```python
from build123d import *

# Parameters (mm, degrees)
SKETCH1_W                      = 276.225
SKETCH1_H                      = 98.425
BOSS_EXTRUDE1_DEPTH            = 6.35
F_5_16_0_332_DOWEL_HOLE1_D     = 7.9375
F_5_16_0_332_DOWEL_HOLE1_DEPTH = 6.35
SKETCH5_W                      = 12.7
SKETCH5_H                      = 12.7
CUT_EXTRUDE1_DEPTH             = 7.35
FILLET1_R                      = 3.175
FILLET2_R                      = 6.35
F_1_4_0_2500_DOWEL_HOLE1_D     = 6.35
F_1_4_0_2500_DOWEL_HOLE1_DEPTH = 6.35


with BuildPart() as part:
    # Sketch1 → Boss-Extrude1 (new body)
    with BuildSketch(Plane(origin=(0, 0, 0), x_dir=(1, 0, 0), z_dir=(0, 1, 0))):
        Rectangle(SKETCH1_W, SKETCH1_H)
    extrude(amount=BOSS_EXTRUDE1_DEPTH)

    # 5/16 (0.332) Dowel Hole1
    with Locations(Plane(origin=(0, 6.35, 0), x_dir=(1, 0, 0), z_dir=(0, 1, 0))):
        with Locations((-93.6625, 0), (93.6625, 0)):
            Hole(F_5_16_0_332_DOWEL_HOLE1_D / 2, depth=F_5_16_0_332_DOWEL_HOLE1_DEPTH)

    # Sketch5 → Cut-Extrude1 (cut, through all)
    with BuildSketch(Plane(origin=(0, 6.35, 0), x_dir=(1, 0, 0), z_dir=(0, 1, 0))):
        with Locations((-131.7625, 0)):
            Rectangle(SKETCH5_W, SKETCH5_H)
        with Locations((131.7625, 0)):
            Rectangle(SKETCH5_W, SKETCH5_H)
    extrude(amount=-CUT_EXTRUDE1_DEPTH, mode=Mode.SUBTRACT)

    # Fillet1
    fillet1_edges = [part.edges().sort_by_distance(p)[0] for p in [
        (-125.4125, 3.175, -6.35),
        (-125.4125, 3.175, 6.35),
        (125.4125, 3.175, 6.35),
        (125.4125, 3.175, -6.35),
    ]]
    fillet(fillet1_edges, radius=FILLET1_R)

    # Fillet2
    fillet2_edges = [part.edges().sort_by_distance(p)[0] for p in [
        (-138.1125, 3.175, 6.35),
        (-138.1125, 3.175, -6.35),
        (138.1125, 3.175, -6.35),
        (138.1125, 3.175, 6.35),
        (-138.1125, 3.175, -49.2125),
        (138.1125, 3.175, -49.2125),
        (138.1125, 3.175, 49.2125),
        (-138.1125, 3.175, 49.2125),
    ]]
    fillet(fillet2_edges, radius=FILLET2_R)

    # 1/4 (0.2500) Dowel Hole1
    with Locations(Plane(origin=(0, 6.35, 0), x_dir=(1, 0, 0), z_dir=(0, 1, 0))):
        with Locations((-57.15, 0), (-31.75, 0), (31.75, 0), (57.15, 0), (-49.493351826, 28.575), (-27.49630657, 15.875), (-27.49630657, -15.875), (-49.493351826, -28.575), (27.49630657, 15.875), (49.493351826, 28.575), (49.493351826, -28.575), (27.49630657, -15.875)):
            Hole(F_1_4_0_2500_DOWEL_HOLE1_D / 2, depth=F_1_4_0_2500_DOWEL_HOLE1_DEPTH)


solid = part.part
```
Here's how the part is built. I have some questions about the finished solid (model axes, mm). A direction names the side the tool comes from. Coordinates: 2 decimals unless noted, no trailing zeros. Order: outer loops, then holes, each group sorted by start corner. A loop starts at its lowest first (then second) coordinate and runs counter-clockwise, first axis right, second up. Notation, with made-up numbers: M -0.75,45 L 21.25,45 A17 cw 21.25,55 Z; hole C 43,28.5 d1. An arc over 180 degrees is marked long. Answer as a JSON object with one key per item and string values. Group by question number.
(1) For pin 1 (2 mm diameter, centred on x = -91.5, z = -36, fed in from -Y); pin 2 (1.9 mm diameter, centred on y = 2.5, z = -1, fed in from +X); pin 3 (5 mm diameter, centred on x = 49.49, z = 28.58, fed in from +Y), each with a flat end and sliding along its axis, tell me the tip position at first contact or that it passes through.
(2) If we mould it in two halves opening along Z, with no side actions, what happens to faces 1 (the face through (-2, 0, -1)), 2 (the face through (46.465, 3.131, 27.621)), 3 (the face through (-50.96, 3.13, -25.76)), 4 (the face through (136.203, 3.219, -47.402))? For each: released by +Z, released by -Z, zero draft, split by the parting line, or undercut.
(3) Which directions (+Z, -Z, +X, -X, +Y, -Y) give clear straight access to the entire face, cutting with the end or side of a thin tool? Please do faces 5 (the face through (-136.2, 3.13, -8.16)), 6 (the face through (46.56, 3.13, -27.36)), 7 (the face through (136.3, 3.13, 8.26)).
(4) I need wall thicknesses on probe 1 along X at (y, z) = (5.75, 17); probe 2 along Z at (x, y) = (49, 0.5); probe 3 along X at (y, z) = (4, -43). Which ranges of each line are inside material? Lowest first, please.
(5) Suppose I cut it at C-C, the plane x = -93.5. Please give me the cut outline in (y, z), then the cut area to 3 significant figures.
(6) Suppose I cut it at A-A, the plane z = 0. State how many separate pieces and enclosed holes the cut face has, then the cut area to 3 significant figures.
Values found:
{
 "1": {"pin 1": "stops at y = 0", "pin 2": "stops at x = 125.41", "pin 3": "passes through"},
 "2": {"face 1": "zero draft", "face 2": "undercut", "face 3": "undercut", "face 4": "released by -Z"},
 "3": {"face 5": "-X, +Y, -Y", "face 6": "+Y, -Y", "face 7": "+X, +Y, -Y"},
 "4": {"probe 1": "x = -138.11 to -30.47, -24.53 to 24.53, 30.47 to 138.11", "probe 2": "z = -49.21 to -31.71, -25.44 to 25.44, 31.71 to 49.21", "probe 3": "x = -138.11 to 138.11"},
 "5": {"outline": "M 0,-49.21 L 6.35,-49.21 L 6.35,-3.97 L 0,-3.97 Z; M 0,3.97 L 6.35,3.97 L 6.35,49.21 L 0,49.21 Z", "area": "575 mm^2"},
 "6": {"separate pieces": "7", "enclosed holes": "0", "area": "1,330 mm^2"}
}
